```python
from build123d import *

# Parameters (mm, degrees)
SKETCH_2_R          = 1.6
CUT_EXTRUDE_1_DEPTH = 36.114099732
SKETCH_5_R          = 4
SKETCH_5_R_2        = 3.326438837
EXTRUDE_1_DEPTH     = 0.3
EXTRUDE_START       = 5
SKETCH_6_R          = 14
SKETCH_6_R_2        = 3.326438837
SKETCH_6_R_3        = 1.6
EXTRUDE_2_DEPTH     = 5
CUT_EXTRUDE_START   = 1
SKETCH_3_R          = 3.25
CUT_EXTRUDE_5_DEPTH = 37.114099894
CUT_EXTRUDE_START_2 = -4
SKETCH_7_R          = 4
SKETCH_7_R_2        = 3.326438837
CUT_EXTRUDE_6_DEPTH = 4
SKETCH_8_W          = 12
SKETCH_8_H          = 0.8
CUT_EXTRUDE_7_DEPTH = 30


with BuildPart() as part:
    # 草图1 → 旋转1 (revolve)
    with BuildSketch(Plane.XY, mode=Mode.PRIVATE) as revolve_1_sk:
        Polygon((4, 29), (4, 0), (14, 0), (14, 0.1), (7, 29), align=None)
    revolve(revolve_1_sk.sketch.rotate(Axis((0, 0, 0), (0, 1, 0)), 90), axis=Axis((0, 0, 0), (0, 1, 0)))

    # 草图2 → 切除-拉伸1 (cut, through all)
    with BuildSketch(Plane.XZ):
        with Locations(Location((8, 0, 0), (0, 0, 270))):
            Circle(SKETCH_2_R)
        with Locations(Location((0, 9.5, 0), (0, 0, 270))):
            Circle(SKETCH_2_R)
        with Locations(Location((0, -9.5, 0), (0, 0, 270))):
            Circle(SKETCH_2_R)
        with Locations(Location((-8, 0, 0), (0, 0, 270))):
            Circle(SKETCH_2_R)
    extrude(amount=-CUT_EXTRUDE_1_DEPTH, mode=Mode.SUBTRACT)

    # 草图5 → 凸台-拉伸1 (add)
    with BuildSketch(Plane.XZ):
        with Locations(Location((0, 0, 0), (0, 0, 270))):
            Circle(SKETCH_5_R)
        with Locations(Location((0, 0, 0), (0, 0, 270))):
            Circle(SKETCH_5_R_2, mode=Mode.SUBTRACT)
    extrude(amount=-EXTRUDE_1_DEPTH)

    # 草图6 → 凸台-拉伸2 (add)
    with BuildSketch(Plane.XZ.offset(EXTRUDE_START)):
        with Locations(Location((0, 0, 0), (0, 0, 270))):
            Circle(SKETCH_6_R)
        with Locations(Location((0, 0, 0), (0, 0, 270))):
            Circle(SKETCH_6_R_2, mode=Mode.SUBTRACT)
        with Locations(Location((0, 9.5, 0), (0, 0, 270))):
            Circle(SKETCH_6_R_3, mode=Mode.SUBTRACT)
        with Locations(Location((-8, 0, 0), (0, 0, 270))):
            Circle(SKETCH_6_R_3, mode=Mode.SUBTRACT)
        with Locations(Location((8, 0, 0), (0, 0, 270))):
            Circle(SKETCH_6_R_3, mode=Mode.SUBTRACT)
        with Locations(Location((0, -9.5, 0), (0, 0, 270))):
            Circle(SKETCH_6_R_3, mode=Mode.SUBTRACT)
    extrude(amount=-EXTRUDE_2_DEPTH)

    # 草图3 → 切除-拉伸5 (cut, through all)
    with BuildSketch(Plane.XZ.offset(CUT_EXTRUDE_START)):
        with Locations(Location((0, 9.5, 0), (0, 0, 270))):
            Circle(SKETCH_3_R)
        with Locations(Location((8, 0, 0), (0, 0, 270))):
            Circle(SKETCH_3_R)
        with Locations(Location((0, -9.5, 0), (0, 0, 270))):
            Circle(SKETCH_3_R)
        with Locations(Location((-8, 0, 0), (0, 0, 270))):
            Circle(SKETCH_3_R)
    extrude(amount=-CUT_EXTRUDE_5_DEPTH, mode=Mode.SUBTRACT)

    # 草图7 → 切除-拉伸6 (cut)
    with BuildSketch(Plane(origin=(0, 0.3, 0), x_dir=(1, 0, 0), z_dir=(0, 1, 0)).offset(CUT_EXTRUDE_START_2)):
        with Locations(Location((0, 0, 0), (0, 0, 90))):
            Circle(SKETCH_7_R)
        with Locations(Location((0, 0, 0), (0, 0, 90))):
            Circle(SKETCH_7_R_2, mode=Mode.SUBTRACT)
    extrude(amount=CUT_EXTRUDE_6_DEPTH, mode=Mode.SUBTRACT)

    # 草图8 → 切除-拉伸7 (cut)
    with BuildSketch(Plane(origin=(0, 29, 0), x_dir=(1, 0, 0), z_dir=(0, 1, 0))):
        Rectangle(SKETCH_8_W, SKETCH_8_H)
    extrude(amount=-CUT_EXTRUDE_7_DEPTH, mode=Mode.SUBTRACT)


solid = part.part
```
The listing builds one solid part. Answer for the finished solid, in the listing's coordinates (mm). A direction names the side the tool comes from. Give positions to 0.01 mm unless a question says otherwise; leave off trailing zeros. Write each loop counter-clockwise with the first axis right and the second up, starting at its lowest first coordinate (ties: lowest second). Pieces come first, ordered by that corner, then holes. Notation, with made-up numbers: (-32, 4.5) - (14, 4.5) arc R21 ccw to (14, 23.5) - close; hole circle Ø4 at (42.25, 88.5). An arc over 180 degrees is marked (long way). Use one line per item in the form item = value. Start each with the question number.
1) Find section A-A on x = 0. Determine the outline of the cut face in (y, z), plus the area to 3 significant figures.
2) Find section C-C on y = 14. Determine the outline of the cut face in (x, z).
3) Consider line 1 along Y through (x, z) = (7.25, -3); line 2 along Z through (x, y) = (2, 17); line 3 along Z through (x, y) = (10.5, 2.5). Determine where each line is inside the solid, lowest interval first. Write a range as from..to.
4) Flat-ended cylindrical pins translate along their axes: pin 1 Ø10.5 at (x, z) = (-8, 0) entering from +Y; pin 2 Ø6 at (x, z) = (8, 0) entering from +Y; pin 3 Ø4 at (y, z) = (17.5, -5.5) entering from +X; pin 4 Ø6 at (x, y) = (-8, 14.5) entering from -Z. Find the tip coordinate at first contact, or state that the pin passes through.
5) Find section B-B on y = 7.5. Determine the outline of the cut face in (x, z).
6) A tool of negligible diameter and unlimited length cuts with its end or side. For faces 1 (the face through (-2, -3.7, 3)), 2 (the face through (-0.1, 29, 4.3)), from which of +Z, -Z, +X, -X, +Y, -Y can it reach the whole face along a straight path? Write none if from no direction.
Geometry results:
q1.outline = (-5, -14) - (0.1, -14) - (5.26, -12.75) - (-1, -12.75) - (-1, -11.1) - (-5, -11.1) - close; (-5, -7.9) - (-1, -7.9) - (-1, -6.25) - (29, -6.25) - (29, -4) - (-3.7, -4) - (-3.7, -3.33) - (-5, -3.33) - close; (-5, 3.33) - (-3.7, 3.33) - (-3.7, 4) - (29, 4) - (29, 6.25) - (-1, 6.25) - (-1, 7.9) - (-5, 7.9) - close; (-5, 11.1) - (-1, 11.1) - (-1, 12.75) - (5.26, 12.75) - (0.1, 14) - (-5, 14) - close
q1.area = 200 mm2
q2.outline = (-10.41, -2.18) arc R10.63 ccw to (-3.19, -10.14) arc R3.25 cw (long way) to (3.19, -10.14) arc R10.63 ccw to (10.41, -2.18) arc R3.25 cw to (4.77, -0.4) - (3.98, -0.4) arc R4 cw to (-3.98, -0.4) - (-4.77, -0.4) arc R3.25 cw to start; (-10.41, 2.18) arc R3.25 cw to (-4.77, 0.4) - (-3.98, 0.4) arc R4 cw to (3.98, 0.4) - (4.77, 0.4) arc R3.25 cw to (10.41, 2.18) arc R10.63 ccw to (3.19, 10.14) arc R3.25 cw (long way) to (-3.19, 10.14) arc R10.63 ccw to start
q3.line_1 = -5..-1
q3.line_2 = -6.94..-3.46, 3.46..6.94
q3.line_3 = -8.36..-2.08, 2.08..8.36
q4.pin_1 = 29
q4.pin_2 = -1
q4.pin_3 = 9.29
q4.pin_4 = -9.44
q5.outline = (-2.03, -12.04) arc R3.25 cw (long way) to (2.03, -12.04) arc R12.21 ccw to (2.03, 12.04) arc R3.25 cw (long way) to (-2.03, 12.04) arc R12.21 ccw to start; hole (-4.77, -0.4) - (-3.98, -0.4) arc R4 ccw to (3.98, -0.4) - (4.77, -0.4) arc R3.25 ccw (long way) to (4.77, 0.4) - (3.98, 0.4) arc R4 ccw to (-3.98, 0.4) - (-4.77, 0.4) arc R3.25 ccw (long way) to start
q6.face_1 = +Y
q6.face_2 = +Z, -Z, +X, -X, +Y
